Geometry check sheet. Reference: the model listing, model coordinates, mm. A direction names the side the tool comes from. Coordinates: 2 decimals unless noted, no trailing zeros. Loops run counter-clockwise (first coordinate to the right, second up) from the corner with the lowest first, then second, coordinate; pieces in that order, holes last.
from build123d import *

# Parameters (mm, degrees)
SKETCH001_R      = 1.5
EXTRUDE001_DEPTH = 10
EXTRUDE_DEPTH    = 3


with BuildPart() as extrude001:
    # Sketch001 (on Face8 of Extrude) → Extrude001 (new body)
    with BuildSketch(Plane.XY.offset(3)):
        with Locations((-23.730994, 38.396749)):
            Circle(SKETCH001_R)
        Polygon((-65.179059, 2), (-54.13242, 17.905464), (-31.230994, 2), align=None)
        Polygon((-31.230994, 5.652561), (-52.421109, 20.369488), (-31.230994, 50.88), align=None)
        with BuildLine():
            Line((-28.230994, 38.396749), (-28.230994, 2))
            Line((-28.230994, 2), (-1.236094, 2))
            Line((-1.236094, 2), (-1.236094, 50.88))
            Line((-19.230994, 50.88), (-1.236094, 50.88))
            Line((-19.230994, 50.88), (-19.230994, 38.396747))
            ThreePointArc((-28.230994, 38.396749), (-23.730995, 33.896749), (-19.230994, 38.396747))
        make_face()
    extrude(amount=-EXTRUDE001_DEPTH)


with BuildPart() as part_mirroring:
    # Part__Mirroring: instance of Extrude001
    add(extrude001.part.mirror(Plane(origin=(0, 0, 0), x_dir=(1, 0, 0), z_dir=(0, 1, 0))))


with BuildPart() as part_mirroring001:
    # Part__Mirroring001: instance of Part__Mirroring
    add(part_mirroring.part.mirror(Plane(origin=(0, 0, 0), x_dir=(0, -1, 0), z_dir=(1, 0, 0))))


with BuildPart() as part_mirroring002:
    # Part__Mirroring002: instance of Extrude001
    add(extrude001.part.mirror(Plane(origin=(0, 0, 0), x_dir=(0, -1, 0), z_dir=(1, 0, 0))))


with BuildPart() as cut003:
    # Sketch → Extrude (new body)
    with BuildSketch(Plane.XY):
        Polygon((-32.8, 53.88), (32.8, 53.88), (70.220657, 0), (32.8, -53.88), (-32.8, -53.88), (-70.220657, 0), align=None)
    extrude(amount=EXTRUDE_DEPTH)

    # Cut: cut Part__Mirroring002
    add(part_mirroring002.part, mode=Mode.SUBTRACT)

    # Cut001: cut Extrude001
    add(extrude001.part, mode=Mode.SUBTRACT)

    # Cut002: cut Part__Mirroring001
    add(part_mirroring001.part, mode=Mode.SUBTRACT)

    # Cut003: cut Part__Mirroring
    add(part_mirroring.part, mode=Mode.SUBTRACT)


solid = cut003.part
1) Access from +Z, -Z, +X, -X, +Y, -Y to the whole of each face (thin tool, end or side, straight path). Record for faces 1 (the flat face through (-59.733, -9.841, 1.521)), 2 (the flat face through (0, -53.88, 1)).
Data:
face 1: +Z, -Z
face 2: +Z, -Z, +X, -X, -Y
2) Mould release check, pull along Y, two halves, no side actions. Record for faces 3 (the flat face through (28.231, -20, 2)), 4 (the flat face through (0, 0, 0)), 5 (the flat face through (-51.772, 26.563, 1.479)): +Y half, -Y half, draft (parallel to the pull), parting line (faces both ways), or undercut.
Data:
face 3: undercut
face 4: draft
face 5: +Y half
3) Section check B-B on x = -35.5. Record the cut outline in (y, z), and give its area (3 significant figures).
Data:
outline: (-49.99, 0) - (-44.73, 0) - (-44.73, 3) - (-49.99, 3) - close; (-8.62, 0) - (-4.96, 0) - (-4.96, 3) - (-8.62, 3) - close; (-2, 0) - (2, 0) - (2, 3) - (-2, 3) - close; (4.96, 0) - (8.62, 0) - (8.62, 3) - (4.96, 3) - close; (44.73, 0) - (49.99, 0) - (49.99, 3) - (44.73, 3) - close
area: 65.5 mm2
4) Section check A-A on x = 13.5. Record the cut outline in (y, z).
Data:
outline: (-53.88, 0) - (-50.88, 0) - (-50.88, 3) - (-53.88, 3) - close; (-2, 0) - (2, 0) - (2, 3) - (-2, 3) - close; (50.88, 0) - (53.88, 0) - (53.88, 3) - (50.88, 3) - close
5) Section check C-C on y = -14. Record the cut outline in (x, z).
Data:
outline: (-60.5, 0) - (-56.84, 0) - (-56.84, 3) - (-60.5, 3) - close; (-48.51, 0) - (-43.25, 0) - (-43.25, 3) - (-48.51, 3) - close; (-31.23, 0) - (-28.23, 0) - (-28.23, 3) - (-31.23, 3) - close; (-1.24, 0) - (1.24, 0) - (1.24, 3) - (-1.24, 3) - close; (28.23, 0) - (31.23, 0) - (31.23, 3) - (28.23, 3) - close; (43.25, 0) - (48.51, 0) - (48.51, 3) - (43.25, 3) - close; (56.84, 0) - (60.5, 0) - (60.5, 3) - (56.84, 3) - close
6) Depth check by flat-ended pin: pin 1 (0.9 mm diameter, centred on y = 35, z = 1.5, fed in from -X); pin 2 (1.5 mm diameter, centred on y = -21.5, z = 2, fed in from -X); pin 3 (1.8 mm diameter, centred on x = -23.73, y = 38.4, fed in from +Z); pin 4 (1.5 mm diameter, centred on y = -29, z = 1.5, fed in from -X). Enter the tip coordinate at first touch or a pass-through.
Data:
pin 1: stops at x = -46.23
pin 2: stops at x = -55.81
pin 3: passes through
pin 4: stops at x = -50.6
7) Section check D-D on z = 2.25. Count the separate pieces of the cut face and the enclosed holes in it, and give its area (3 significant figures).
Data:
separate pieces: 1
enclosed holes: 16
area: 3,380 mm2
8) Material ranges on probe 1 along Y at (x, z) = (-13, 2.65); probe 2 along Y at (x, z) = (24, 0.7); probe 3 along X at (y, z) = (49, 2.35), recorded low to high.
Data:
probe 1: y = -53.88 to -50.88, -2 to 2, 50.88 to 53.88
probe 2: y = -53.88 to -39.87, -36.92 to -33.9, -2 to 2, 33.9 to 36.92, 39.87 to 53.88
probe 3: x = -36.19 to -32.54, -31.23 to -19.23, -1.24 to 1.24, 19.23 to 31.23, 32.54 to 36.19
